from build123d import *

# Parameters (mm, degrees)
F0_R        = 38.1
F1_DEPTH    = 20.32
F2_R        = 38.1
F3_DEPTH    = 124.46
F5_DEPTH    = 122.682
F6_T2_ANGLE = 179.9999997765
F6_T4_ANGLE = 180.0000002235


# Not quite as in the source:
# - a fillet or chamfer that OpenCascade refuses, or shapes differently, is made with other operations: its cross-section is extruded or revolved along the edge and cut away or added
# - a feature names something its author has since deleted; it is built from what else it names


with BuildPart() as f1:
    # F0 (on Top) → F1 (new body)
    with BuildSketch(Plane.XY):
        Circle(F0_R)
    extrude(amount=F1_DEPTH)

    # F2 (on face) → F3 (join)
    with BuildSketch(Plane.XY.offset(20.32)):
        Circle(F2_R)
    extrude(amount=F3_DEPTH)

    # F4 (on face) → F5 (cut, symmetric)
    with BuildSketch(Plane.XY.offset(144.78)):
        with BuildLine():
            ThreePointArc((-33.8414182484, 0), (0, -33.8414182484), (33.8414182484, 0))
            ThreePointArc((33.8414182484, 0), (0, 33.8414182484), (-33.8414182484, 0))
        make_face()
    extrude(amount=F5_DEPTH, both=True, mode=Mode.SUBTRACT)

    # F6: fillet of radius 5.08 on 1 edges, made by hand

    # F6_s1 → F6_t2 (revolve, cut)
    with BuildSketch(Plane.XZ):
        with BuildLine():
            ThreePointArc((38.1, 139.7668500859), (36.8916407828, 143.0557401189), (33.8414182484, 144.78))
            Line((33.8414182484, 144.78), (38.1, 144.78))
            Line((38.1, 144.78), (38.1, 139.7668500859))
        make_face()
    revolve(axis=Axis((0, 0, 144.78), (0, 0, 1)), revolution_arc=F6_T2_ANGLE, mode=Mode.SUBTRACT)

    # F6_s3 → F6_t4 (revolve, cut)
    with BuildSketch(Plane.XZ):
        with BuildLine():
            ThreePointArc((-38.1, 139.7668500859), (-36.8916407828, 143.0557401189), (-33.8414182484, 144.78))
            Line((-33.8414182484, 144.78), (-38.1, 144.78))
            Line((-38.1, 144.78), (-38.1, 139.7668500859))
        make_face()
    revolve(axis=Axis((0, 0, 144.78), (0, 0, 1)), revolution_arc=F6_T4_ANGLE, mode=Mode.SUBTRACT)


solid = f1.part
The listing builds one solid part. Answer for the finished solid, in the listing's coordinates (mm). Round coordinates to 2 decimals unless told otherwise and drop trailing zeros. Order: outer loops, then holes, each group sorted by start corner. A loop starts at its lowest first (then second) coordinate and runs counter-clockwise, first axis right, second up. Notation, with made-up numbers: (-5.75, 88) -> (41.25, 88) arc R30 cw to (41.25, 120) -> close; hole circle Ø11 at (-13, 48.5). An arc over 180 degrees is marked (long way). Write each question's results on one line, items separated by ' | '. Start each with the question number.
Q1. Find section B-B (x = 0). Determine the outline of the cut face in (y, z).
Q2. Each of these flat-tipped pins is pushed along its axis until it touches: pin 1 (1.5 mm diameter, centred on y = 18, z = 89.5, fed in from -X); pin 2 (1.5 mm diameter, centred on x = 0.5, y = -15, fed in from +Z); pin 3 (8 mm diameter, centred on y = -28, z = 91, fed in from +X). Where does it stop, or does it pass through?
Q3. Straight lines are drawn through the part: probe 1 along Y at (x, z) = (0, 117); probe 2 along Z at (x, y) = (-8, 28); probe 3 along X at (y, z) = (22.5, 45.5). For each, find the intervals that lie inside material, in ascending order. Write a range as from..to.
Q4. Find section A-A (z = 75.5). Determine the outline of the cut face in (x, y).
Q5. The mould has two halves that part along X. Classify faces 1 (the flat face through (-1, 1, 0)), 2 (the cylindrical face through (36.34, 11.44, 68.91)), 3 (the flat face through (0, 0, 22.098)): pulls with the +X half, pulls with the -X half, needs draft (parallel to the pull), parting line crosses it, or undercut.
Worked answers:
1) outline: (-38.1, 0) -> (38.1, 0) -> (38.1, 139.77) arc R5.08 ccw to (33.84, 144.78) -> (33.84, 22.1) -> (-33.84, 22.1) -> (-33.84, 144.78) arc R5.08 ccw to (-38.1, 139.77) -> close
2) pin 1: stops at x = -33.97 | pin 2: stops at z = 22.1 | pin 3: stops at x = 29.59
3) probe 1: y = -38.1..-33.84, 33.84..38.1 | probe 2: z = 0..22.1 | probe 3: x = -30.75..-25.28, 25.28..30.75
4) outline: circle Ø76.2 at (0, 0); hole circle Ø67.68 at (0, 0)
5) face 1: needs draft | face 2: parting line crosses it | face 3: undercut
